Could you check a few things on this model? Use its own coordinates, in mm. Face numbers are marked on the shaded views. A direction names the side the tool comes from. Round coordinates to 2 decimals unless told otherwise and drop trailing zeros. Write each loop counter-clockwise with the first axis right and the second up, starting at its lowest first coordinate (ties: lowest second). Pieces come first, ordered by that corner, then holes.
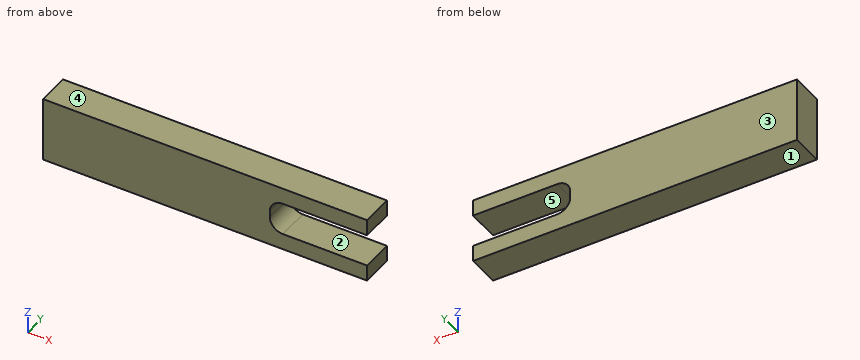
```python
from build123d import *

# Parameters (mm, degrees)
CROQUIS1_W              = 50
CROQUIS1_H              = 10
SALIENTE_EXTRUIR1_DEPTH = 2.5
CORTAR_EXTRUIR1_DEPTH   = 52.23475383


with BuildPart() as part:
    # Croquis1 → Saliente-Extruir1 (new, symmetric)
    with BuildSketch(Plane(origin=(0, 0, 0), x_dir=(1, 0, 0), z_dir=(0, 1, 0))):
        with Locations((25, 5)):
            Rectangle(CROQUIS1_W, CROQUIS1_H)
    extrude(amount=SALIENTE_EXTRUIR1_DEPTH, both=True)

    # Croquis2 → Cortar-Extruir1 (cut, through all)
    with BuildSketch(Plane(origin=(0, 2.5, 0), x_dir=(1, 0, 0), z_dir=(0, 1, 0))):
        with BuildLine():
            Line((50, 7.5), (37, 7.5))
            ThreePointArc((37, 7.5), (35.585786438, 6.914213562), (35, 5.5))
            Line((35, 5.5), (35, 4.5))
            ThreePointArc((35, 4.5), (35.585786438, 3.085786438), (37, 2.5))
            Line((37, 2.5), (50, 2.5))
            Line((50, 2.5), (50, 7.5))
        make_face()
    extrude(amount=-CORTAR_EXTRUIR1_DEPTH, mode=Mode.SUBTRACT)


solid = part.part
```
Q1. Imagine slicing it at C-C, the plane z = -7. Write out the boundary of the cut face in (x, y).
Q2. On a 3-axis mill with a long thin cutter (end or side, diameter ignored), from which of +Z, -Z, +X, -X, +Y, -Y can I reach the whole of each face in a straight line? I mean the marked faces 1 and 2. Say none if no direction works.
Q3. If I drill on L1, parallel to Z at x = 41.5, y = 0.3; L2, parallel to X at y = -1, z = -5; L3, parallel to X at y = 1.8, z = -7, over which ranges is the centre line in solid material (lowest first)?
Q4. Imagine slicing it at A-A, the plane x = 39. Write out the boundary of the cut face in (y, z).
Q5. We'd pull the mould along Z, two halves only. Please class the marked faces 3, 4 and 5: pulls with the +Z half, pulls with the -Z half, needs draft (parallel to the pull), parting line crosses it, or undercut.
Q6. I'm going to push flat-ended pins straight in: pin 1 Ø1.5 at (y, z) = (0, -2) entering from -X; pin 2 Ø0.8 at (y, z) = (-1, -5) entering from +X. Where does each tip first touch, or does it pass through?
Q7. Imagine slicing it at B-B, the plane y = -2. Write out the boundary of the cut face in (x, z), then the cut area to 3 significant figures.
Q8. Imagine slicing it at D-D, the plane z = -3.75. Write out the boundary of the cut face in (x, y), then the cut area to 3 significant figures.
Results found:
1. outline: (0, -2.5) - (35.68, -2.5) - (35.68, 2.5) - (0, 2.5) - close
2. face 1: -Z, +X, -X, +Y, -Y
2. face 2: +X, +Y, -Y
3. L1: z = -10 to -7.5, -2.5 to 0
3. L2: x = 0 to 35
3. L3: x = 0 to 35.68
4. outline: (-2.5, -10) - (2.5, -10) - (2.5, -7.5) - (-2.5, -7.5) - close; (-2.5, -2.5) - (2.5, -2.5) - (2.5, 0) - (-2.5, 0) - close
5. face 3: needs draft
5. face 4: pulls with the +Z half
5. face 5: undercut
6. pin 1: stops at x = 0
6. pin 2: stops at x = 35
7. outline: (0, -10) - (50, -10) - (50, -7.5) - (37, -7.5) arc R2 cw to (35, -5.5) - (35, -4.5) arc R2 cw to (37, -2.5) - (50, -2.5) - (50, 0) - (0, 0) - close
7. area: 427 mm2
8. outline: (0, -2.5) - (35.15, -2.5) - (35.15, 2.5) - (0, 2.5) - close
8. area: 176 mm2
